Part print with two shaded views. Sizes in mm from the minimum x, y, z corner. A direction names the side the tool comes from. Give positions to 0.01 mm unless a question says otherwise; leave off trailing zeros. Write each loop counter-clockwise with the first axis right and the second up, starting at its lowest first coordinate (ties: lowest second). Pieces come first, ordered by that corner, then holes. Notation, with made-up numbers: M 54.5,44 L 88.5,44 A23 cw 88.5,75 Z; hole C -34.5,-29 d7. An arc over 180 degrees is marked long. Return JSON: item names as keys, results as strings. Group by question number.
Q1. Band-saw the part on B-B, the plane z = 43.5. Give the cut face in (x, y).
Q2. Flat gauge pins, fed straight in: pin 1 Ø10 at (x, y) = (50.8, 82.55) entering from -Z; pin 2 Ø12 at (x, y) = (38.5, 13.5) entering from +Z (3 decimals); pin 3 Ø22 at (x, y) = (39, 11.5) entering from +Z; pin 4 Ø12.5 at (x, z) = (29, 37.5) entering from -Y. Where does each tip first touch, or does it go through?
Q3. Wall check: probe 1 along X at (y, z) = (82, 26); probe 2 along Y at (x, z) = (31.75, 18.5) (3 decimals); probe 3 along X at (y, z) = (83.5, 31.5). Give the ranges that are in metal, low to high.
Q4. Tool access for the marked faces 4, 5 and 6: list every direction of +Z, -Z, +X, -X, +Y, -Y with a clear straight run to the whole face (end or side of a thin tool).
Q5. Band-saw the part on A-A, the plane y = 82.55. Give the cut face in (x, z) (3 decimals), then the cut area to 3 significant figures.
Q6. Pull direction Y, two halves, no side cores. Call the marked faces 1, 2 and 3: +Y half, -Y half, draft (parallel to the pull), parting line (faces both ways), or undercut.
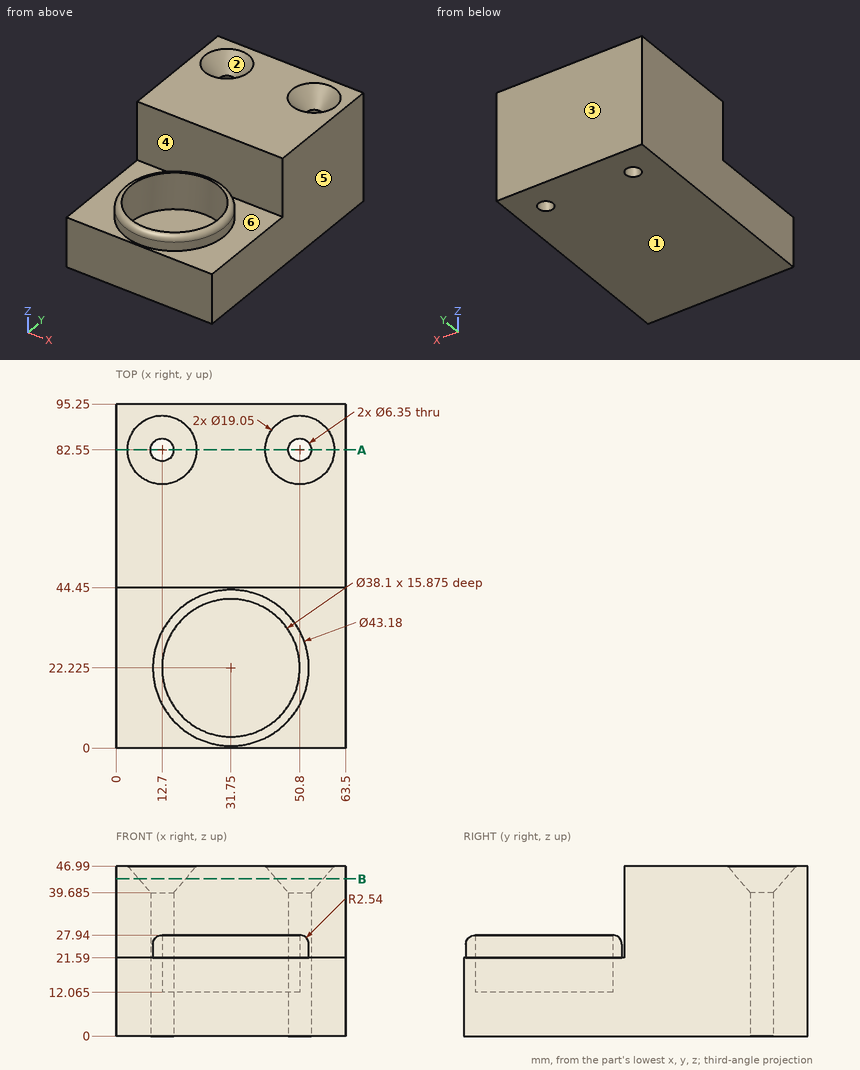
From the geometry:
{
 "1": {"outline": "M 0,44.45 L 63.5,44.45 L 63.5,95.25 L 0,95.25 Z; hole C 12.7,82.55 d12.98; hole C 50.8,82.55 d12.98"},
 "2": {"pin 1": "stops at z = 0", "pin 2": "stops at z = 12.065", "pin 3": "stops at z = 27.94", "pin 4": "stops at y = 44.45"},
 "3": {"probe 1": "x = 0 to 9.57, 15.83 to 47.67, 53.93 to 63.5", "probe 2": "y = 0 to 3.175, 41.275 to 95.25", "probe 3": "x = 0 to 9.67, 15.73 to 47.77, 53.83 to 63.5"},
 "4": {"face 4": "+Z, +X, -X", "face 5": "+Z, -Z, +X, +Y, -Y", "face 6": "+Z"},
 "5": {"outline": "M 0,0 L 9.525,0 L 9.525,39.685 L 3.175,46.99 L 0,46.99 Z; M 15.875,0 L 47.625,0 L 47.625,39.685 L 41.275,46.99 L 22.225,46.99 L 15.875,39.685 Z; M 53.975,0 L 63.5,0 L 63.5,46.99 L 60.325,46.99 L 53.975,39.685 Z", "area": "2,290 mm^2"},
 "6": {"face 1": "draft", "face 2": "undercut", "face 3": "+Y half"}
}
